Here's the drawing with two shaded views (mm, measured from the low corner). I have some questions. A direction names the side the tool comes from. Round coordinates to 2 decimals unless told otherwise and drop trailing zeros. Order: outer loops, then holes, each group sorted by start corner. A loop starts at its lowest first (then second) coordinate and runs counter-clockwise, first axis right, second up.
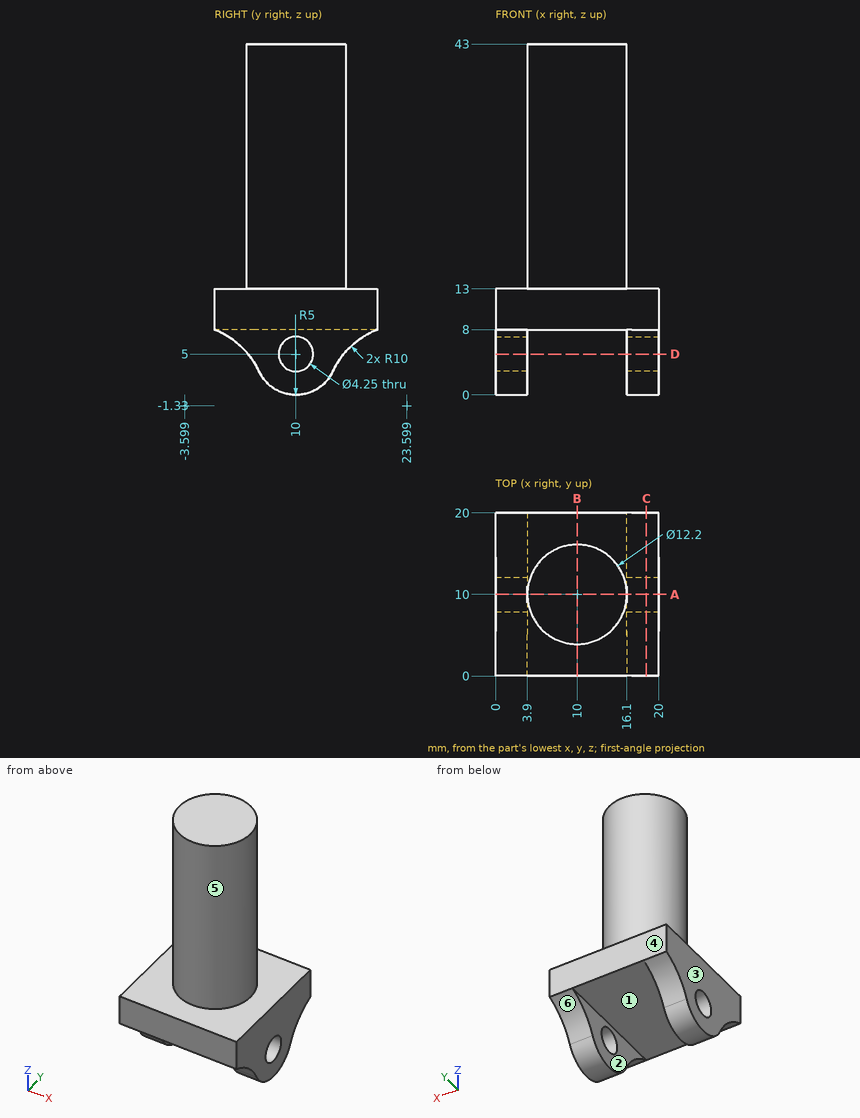
1. If we section it at B-B, the plane x = 10: Write out the boundary of the cut face in (y, z).
Evaluation:
outline: (0, 8) - (20, 8) - (20, 13) - (16.1, 13) - (16.1, 43) - (3.9, 43) - (3.9, 13) - (0, 13) - close
2. If we section it at C-C, the plane x = 18.5: Write out the boundary of the cut face in (y, z) (3 decimals).
Evaluation:
outline: (0, 8) arc R10 cw to (5.467, 2.89) arc R5 ccw to (14.533, 2.89) arc R10 cw to (20, 8) - (20, 13) - (0, 13) - close; hole circle Ø4.25 at (10, 5)
3. If we section it at A-A, the plane y = 10: Write out the boundary of the cut face in (x, z) (3 decimals), and give its area (3 significant figures).
Evaluation:
outline: (0, 0) - (3.9, 0) - (3.9, 2.875) - (0, 2.875) - close; (0, 7.125) - (3.9, 7.125) - (3.9, 8) - (16.1, 8) - (16.1, 7.125) - (20, 7.125) - (20, 13) - (16.1, 13) - (16.1, 43) - (3.9, 43) - (3.9, 13) - (0, 13) - close; (16.1, 0) - (20, 0) - (20, 2.875) - (16.1, 2.875) - close
area: 495 mm2
4. I'm going to push flat-ended pins straight in: P1, Ø12, axis at y = 18, z = 38.5, coming from the +X side; P2, Ø3.5, axis at x = 7, y = 10.5, coming from the -Z side; P3, Ø8, axis at y = 14.5, z = 20, coming from the -X side. Where does each tip first touch, or does it pass through?
Evaluation:
P1: stops at x = 15.76
P2: stops at z = 8
P3: stops at x = 3.92
5. On a 3-axis mill with a long thin cutter (end or side, diameter ignored), from which of +Z, -Z, +X, -X, +Y, -Y can I reach the whole of each face in a straight line? I mean the marked faces 5 and 6. Say none if no direction works.
Evaluation:
face 5: +Z
face 6: -Z, +X, -X, +Y
6. If we section it at D-D, the plane z = 5: Write out the boundary of the cut face in (x, y) (1 decimal).
Evaluation:
outline: (0, 4.1) - (3.9, 4.1) - (3.9, 7.9) - (0, 7.9) - close; (0, 12.1) - (3.9, 12.1) - (3.9, 15.9) - (0, 15.9) - close; (16.1, 4.1) - (20, 4.1) - (20, 7.9) - (16.1, 7.9) - close; (16.1, 12.1) - (20, 12.1) - (20, 15.9) - (16.1, 15.9) - close
7. If we mould it in two halves opening along X, with no side actions, what happens to the marked faces 1, 2, 3 and 4? For each: released by +X, released by -X, zero draft, split by the parting line, or undercut.
Evaluation:
face 1: undercut
face 2: undercut
face 3: released by -X
face 4: zero draft
8. I need wall thicknesses on probe 1 along X at (y, z) = (3.75, 7); probe 2 along Y at (x, z) = (17.7, 5) (1 decimal); probe 3 along Z at (x, y) = (9.5, 16.5). Which ranges of each line are inside material? Lowest first, please.
Evaluation:
probe 1: x = 0 to 3.9, 16.1 to 20
probe 2: y = 4.1 to 7.9, 12.1 to 15.9
probe 3: z = 8 to 13
